Source: CAD feature listing. Evaluate the final solid. Frame: model axes, mm. A direction names the side the tool comes from. Coordinates: 2 decimals unless noted, no trailing zeros. Loops run counter-clockwise (first coordinate to the right, second up) from the corner with the lowest first, then second, coordinate; pieces in that order, holes last.
Item 1: Section query C-C, the plane x = 15. Return the cut outline in (y, z) (3 decimals), then the cut area to 3 significant figures.
Item 2: Reachability of faces 1 (the flat face through (-9.38, 4.93, 15.947)), 2 (the flat face through (18.5, 5, 0)), 3 (the flat face through (-9.12, 4.93, -16.096)), 4 (the flat face through (-11, 0, -16)) from +Z, -Z, +X, -X, +Y, -Y: full face, straight path, thin tool, end or side. Return the list, or none.
Item 3: Pull-direction query (Z, two-part tool) for faces 5 (the flat face through (-6, 10, 16)), 6 (the cylindrical face through (-15.24, 2.11, -6.32)), 7 (the flat face through (9.38, 4.93, -15.947)); classes: +Z half, -Z half, draft (parallel to the pull), parting line (faces both ways), or undercut.
Item 4: Section query B-B, the plane z = -6. Return the cut outline in (x, y), then the cut area to 3 significant figures.
Item 5: Section query D-D, the plane z = 18.5. Return the cut outline in (x, y).
Item 6: Section query A-A, the plane y = 3.75. Return the cut outline in (x, z), then the cut area to 3 significant figures.
Item 7: Pin query (flat end, axial travel): pin 1 Ø2 at (x, z) = (-3, -14.5) entering from +Y; pin 2 Ø2 at (x, y) = (2.5, 2) entering from -Z; pin 3 Ø4 at (x, y) = (18, 5) entering from -Z; pin 4 Ø3 at (y, z) = (3.5, 8) entering from +X. Return the tip coordinate at first contact, or that it passes through.
Item 8: Line query: probe 1 along Z at (x, y) = (0, 2.5); probe 2 along X at (y, z) = (0.75, 0); probe 3 along Z at (x, y) = (-7, -4). Output: solid intervals per line, ascending.
Autodesk Fusion 360 part; units mm, degrees
sketch "スケッチ1" plane through (0, 0, 0) normal (0, 1, 0) x (1, 0, 0)
  line L0 (-18.5, -10.681) -> (0, -21.362)
  line L1 (0, -21.362) -> (18.5, -10.681)
  line L2 (18.5, -10.681) -> (18.5, 10.681)
  line L3 (18.5, 10.681) -> (0, 21.362)
  line L4 (0, 21.362) -> (-18.5, 10.681)
  line L5 (-18.5, 10.681) -> (-18.5, -10.681)
  curve L6
  line L7 (1.75, 0) -> (22.5, 0)
  dimension "d7" = 37
extrude "押し出し1" add sketch "スケッチ1" along normal blind 10
sketch "スケッチ3" plane through (0, 0, 0) normal (0, 1, 0) x (1, 0, 0)
  circle A0 centre (0, 0) radius 24
  dimension "d8" = 48
extrude "押し出し3" add sketch "スケッチ3" against normal blind 6
sketch "スケッチ4" plane through (0, 0, 0) normal (0, 1, 0) x (-1, 0, 0)
  circle A0 centre (0, 0) radius 24
  line L0 (18.5, -10.681) -> (0, -21.362)
  line L1 (0, -21.362) -> (-18.5, -10.681)
  line L2 (-18.5, -10.681) -> (-18.5, 10.681)
  line L3 (-18.5, 10.681) -> (0, 21.362)
  line L4 (0, 21.362) -> (18.5, 10.681)
  line L5 (18.5, 10.681) -> (18.5, -10.681)
  circle A1 centre (0, 0) radius 16.5
  dimension "d11" = 33
extrude "押し出し4" cut sketch "スケッチ4" along normal mid plane 32 contours A1
thread "ねじ2"
Verdict:
1. outline: (-6, -18.735) - (0, -18.735) - (0, -12.702) - (10, -12.702) - (10, -6.874) - (-6, -6.874) - close; (-6, 6.874) - (10, 6.874) - (10, 12.702) - (0, 12.702) - (0, 18.735) - (-6, 18.735) - close
1. area: 259 mm2
2. face 1: +Z, -X, +Y
2. face 2: +Z, -Z, +X, +Y
2. face 3: -Z, -X, +Y
2. face 4: +Y
3. face 5: draft
3. face 6: undercut
3. face 7: -Z half
4. outline: (-23.24, -6) - (-15.37, -6) - (-15.37, 10) - (-18.5, 10) - (-18.5, 0) - (-23.24, 0) - close; (15.37, -6) - (23.24, -6) - (23.24, 0) - (18.5, 0) - (18.5, 10) - (15.37, 10) - close
4. area: 157 mm2
5. outline: (-15.29, -6) - (15.29, -6) - (15.29, 0) - (4.96, 0) - (4.96, 10) - (-4.96, 10) - (-4.96, 0) - (-15.29, 0) - close
6. outline: (-18.5, -10.68) - (0, -21.36) - (18.5, -10.68) - (18.5, 10.68) - (0, 21.36) - (-18.5, 10.68) - close; hole circle Ø33 at (0, 0)
6. area: 330 mm2
7. pin 1: passes through
7. pin 2: stops at z = -20.5
7. pin 3: stops at z = -12.12
7. pin 4: stops at x = 18.5
8. probe 1: z = -21.36 to -16.5, 16.5 to 21.36
8. probe 2: x = -18.5 to -16.5, 16.5 to 18.5
8. probe 3: z = -22.96 to -14.94, 14.94 to 22.96
